The figure shows three views and two pictorial views of one solid part (mm, origin at its lowest corner). Answer the questions. Round coordinates to 2 decimals unless told otherwise and drop trailing zeros. Order: outer loops, then holes, each group sorted by start corner. A loop starts at its lowest first (then second) coordinate and runs counter-clockwise, first axis right, second up. Notation, with made-up numbers: (67.5, 43) -> (78.5, 43) arc R17 cw to (78.5, 59) -> close; hole circle Ø1 at (24.25, 19.5). An arc over 180 degrees is marked (long way). One line per item, written item: value. Start each with the question number.
1. Consider line 1 (Y direction, x = 6.5, z = 10.5); line 2 (Z direction, x = 72.5, y = 69); line 3 (Y direction, x = 75, z = 18). Determine where each line is inside the solid, lowest interval first.
2. Section A-A (z = 12.5) is taken. Give the vertices of the cut face in (x, y), then the cut area to 3 significant figures.
3. Flat-ended cylindrical pins translate along their axes: pin 1 Ø1.5 at (x, y) = (23, 43) entering from -Z; pin 2 Ø0.8 at (x, z) = (16, 19) entering from -Y; pin 3 Ø4 at (x, z) = (76.5, 12.5) entering from +Y; pin 4 Ø6 at (y, z) = (57.5, 15) entering from -X. Find the tip coordinate at first contact, or state that the pin passes through.
4. Section C-C (y = 13.5) is taken. Give the vertices of the cut face in (x, z).
5. Section B-B (x = 60) is taken. Give the vertices of the cut face in (y, z).
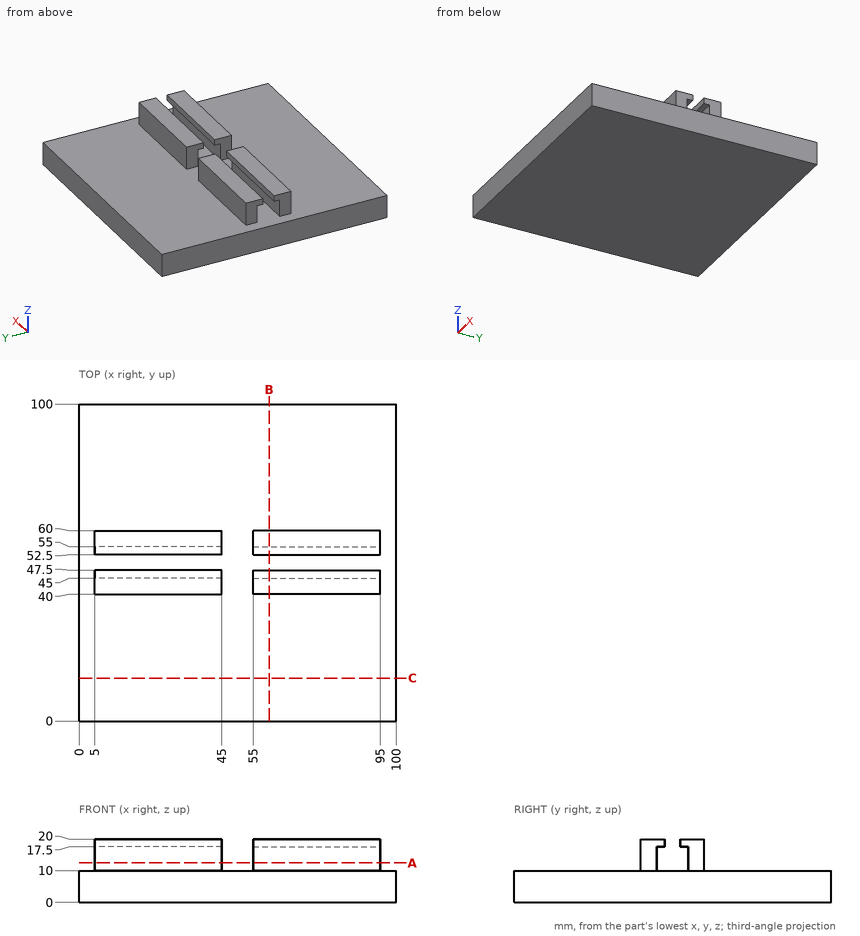
Answer:
1. line 1: 40 to 45, 55 to 60
1. line 2: 0 to 10
1. line 3: 40 to 47.5, 52.5 to 60
2. outline: (5, 40) -> (45, 40) -> (45, 45) -> (5, 45) -> close; (5, 55) -> (45, 55) -> (45, 60) -> (5, 60) -> close; (55, 40) -> (95, 40) -> (95, 45) -> (55, 45) -> close; (55, 55) -> (95, 55) -> (95, 60) -> (55, 60) -> close
2. area: 800 mm^2
3. pin 1: z = 0
3. pin 2: y = 40
3. pin 3: y = 60
3. pin 4: x = 5
4. outline: (0, 0) -> (100, 0) -> (100, 10) -> (0, 10) -> close
5. outline: (0, 0) -> (100, 0) -> (100, 10) -> (60, 10) -> (60, 20) -> (52.5, 20) -> (52.5, 17.5) -> (55, 17.5) -> (55, 10) -> (45, 10) -> (45, 17.5) -> (47.5, 17.5) -> (47.5, 20) -> (40, 20) -> (40, 10) -> (0, 10) -> close
